from build123d import *

# Parameters (mm, degrees)
SKETCH2_W           = 127
SKETCH2_H           = 215.9
BASE_FLANGE1_DEPTH  = 0.7
EDGE_FLANGE4_DEPTH  = 127
EDGE_FLANGE5_DEPTH  = 216.9
EDGE_FLANGE6_DEPTH  = 216.9
EDGE_FLANGE7_DEPTH  = 25.4
EDGE_FLANGE9_DEPTH  = 25.4
EDGE_FLANGE10_DEPTH = 15.4
EDGE_FLANGE11_DEPTH = 15.4
SKETCH76_W          = 12.7
SKETCH76_H          = 12.7
TAB1_DEPTH          = 0.7
SKETCH79_W          = 12.7
SKETCH79_H          = 12.7
TAB2_DEPTH          = 0.7
SKETCH86_R          = 3.15
CUT_EXTRUDE3_DEPTH  = 253.866214627
SKETCH87_W          = 70.35
SKETCH87_H          = 12.7
CUT_EXTRUDE4_DEPTH  = 253.866214627
SKETCH88_R          = 25.4
CUT_EXTRUDE5_DEPTH  = 10
SKETCH90_R          = 25.4
CUT_EXTRUDE6_DEPTH  = 300.389111358


# Sheet-metal steps are written as plain solids
with BuildPart() as part:
    # Sketch2 → Base-Flange1 (new body)
    with BuildSketch(Plane(origin=(0, 0, 0), x_dir=(1, 0, 0), z_dir=(0, 1, 0))):
        Rectangle(SKETCH2_W, SKETCH2_H)
    extrude(amount=-BASE_FLANGE1_DEPTH)

    # Edge-Flange4 section (across the edge) → Edge-Flange4 (add)
    with BuildSketch(Plane(origin=(63.5, 0, -109.95), x_dir=(0, 0, 1), z_dir=(-1, 0, 0))):
        with BuildLine():
            Line((-0.7, 1), (-0.7, 177.8))
            Line((-0.7, 177.8), (0, 177.8))
            Line((0, 177.8), (0, 1))
            ThreePointArc((0, 1), (0.292893219, 0.292893219), (1, 0))
            Line((1, 0), (2, 0))
            Line((2, 0), (2, -0.7))
            Line((2, -0.7), (1, -0.7))
            ThreePointArc((1, -0.7), (-0.202081528, -0.202081528), (-0.7, 1))
        make_face()
    extrude(amount=EDGE_FLANGE4_DEPTH)

    # Edge-Flange5 section (across the edge) → Edge-Flange5 (add)
    with BuildSketch(Plane(origin=(-65.5, 0, -108.95), x_dir=(1, 0, 0), z_dir=(0, 0, 1))):
        with BuildLine():
            Line((-0.7, 1), (-0.7, 177.8))
            Line((-0.7, 177.8), (0, 177.8))
            Line((0, 177.8), (0, 1))
            ThreePointArc((0, 1), (0.292893219, 0.292893219), (1, 0))
            Line((1, 0), (2, 0))
            Line((2, 0), (2, -0.7))
            Line((2, -0.7), (1, -0.7))
            ThreePointArc((1, -0.7), (-0.202081528, -0.202081528), (-0.7, 1))
        make_face()
    extrude(amount=EDGE_FLANGE5_DEPTH)

    # Edge-Flange6 section (across the edge) → Edge-Flange6 (add)
    with BuildSketch(Plane(origin=(65.5, 0, 107.95), x_dir=(-1, 0, 0), z_dir=(0, 0, -1))):
        with BuildLine():
            Line((-0.7, 1), (-0.7, 177.8))
            Line((-0.7, 177.8), (0, 177.8))
            Line((0, 177.8), (0, 1))
            ThreePointArc((0, 1), (0.292893219, 0.292893219), (1, 0))
            Line((1, 0), (2, 0))
            Line((2, 0), (2, -0.7))
            Line((2, -0.7), (1, -0.7))
            ThreePointArc((1, -0.7), (-0.202081528, -0.202081528), (-0.7, 1))
        make_face()
    extrude(amount=EDGE_FLANGE6_DEPTH)

    # Edge-Flange7 section (across the edge) → Edge-Flange7 (add)
    with BuildSketch(Plane(origin=(-65.5, 127, -110.75), x_dir=(0, 0, 1), z_dir=(0, 1, 0))):
        with BuildLine():
            Line((-0.7, 1), (-0.7, 24.7))
            Line((-0.7, 24.7), (0, 24.7))
            Line((0, 24.7), (0, 1))
            ThreePointArc((0, 1), (0.292893219, 0.292893219), (1, 0))
            Line((1, 0), (1.8, 0))
            Line((1.8, 0), (1.8, -0.7))
            Line((1.8, -0.7), (1, -0.7))
            ThreePointArc((1, -0.7), (-0.202081528, -0.202081528), (-0.7, 1))
        make_face()
    extrude(amount=EDGE_FLANGE7_DEPTH)

    # Edge-Flange9 section (across the edge) → Edge-Flange9 (add)
    with BuildSketch(Plane(origin=(65.5, 152.4, -110.75), x_dir=(0, 0, 1), z_dir=(0, -1, 0))):
        with BuildLine():
            Line((-0.7, 1), (-0.7, 24.7))
            Line((-0.7, 24.7), (0, 24.7))
            Line((0, 24.7), (0, 1))
            ThreePointArc((0, 1), (0.292893219, 0.292893219), (1, 0))
            Line((1, 0), (1.8, 0))
            Line((1.8, 0), (1.8, -0.7))
            Line((1.8, -0.7), (1, -0.7))
            ThreePointArc((1, -0.7), (-0.202081528, -0.202081528), (-0.7, 1))
        make_face()
    extrude(amount=EDGE_FLANGE9_DEPTH)

    # Edge-Flange10 section (across the edge) → Edge-Flange10 (add)
    with BuildSketch(Plane(origin=(65.5, 25.4, 120.95), x_dir=(0, 0, -1), z_dir=(0, 1, 0))):
        with BuildLine():
            Line((-0.7, 1), (-0.7, 10))
            Line((-0.7, 10), (0, 10))
            Line((0, 10), (0, 1))
            ThreePointArc((0, 1), (0.292893219, 0.292893219), (1, 0))
            Line((1, 0), (13, 0))
            Line((13, 0), (13, -0.7))
            Line((13, -0.7), (1, -0.7))
            ThreePointArc((1, -0.7), (-0.202081528, -0.202081528), (-0.7, 1))
        make_face()
    extrude(amount=EDGE_FLANGE10_DEPTH)

    # Edge-Flange11 section (across the edge) → Edge-Flange11 (add)
    with BuildSketch(Plane(origin=(-65.5, 40.8, 120.95), x_dir=(0, 0, -1), z_dir=(0, -1, 0))):
        with BuildLine():
            Line((-0.7, 1), (-0.7, 10))
            Line((-0.7, 10), (0, 10))
            Line((0, 10), (0, 1))
            ThreePointArc((0, 1), (0.292893219, 0.292893219), (1, 0))
            Line((1, 0), (13, 0))
            Line((13, 0), (13, -0.7))
            Line((13, -0.7), (1, -0.7))
            ThreePointArc((1, -0.7), (-0.202081528, -0.202081528), (-0.7, 1))
        make_face()
    extrude(amount=EDGE_FLANGE11_DEPTH)

    # Sketch76 → Tab1 (add)
    with BuildSketch(Plane.ZY.offset(66.2)):
        with Locations((114.3, 8.35)):
            Rectangle(SKETCH76_W, SKETCH76_H)
    extrude(amount=-TAB1_DEPTH)

    # Sketch79 → Tab2 (add)
    with BuildSketch(Plane(origin=(66.2, 0, 0), x_dir=(0, 0, -1), z_dir=(1, 0, 0))):
        with Locations((-114.3, 8.35)):
            Rectangle(SKETCH79_W, SKETCH79_H)
    extrude(amount=-TAB2_DEPTH)

    # Sketch86 → Cut-Extrude3 (cut, through all)
    with BuildSketch(Plane(origin=(66.2, 0, 0), x_dir=(0, 0, -1), z_dir=(1, 0, 0))):
        with Locations(Location((-114.3, 8.35, 0), (0, 0, 90))):
            Circle(SKETCH86_R)
    extrude(amount=-CUT_EXTRUDE3_DEPTH, mode=Mode.SUBTRACT)

    # Sketch87 → Cut-Extrude4 (cut, through all)
    with BuildSketch(Plane.ZY.offset(66.2)):
        with Locations((-54.725, 165.1)):
            Rectangle(SKETCH87_W, SKETCH87_H)
        with Locations((53.725, 165.0975)):
            Rectangle(SKETCH87_W, SKETCH87_H)
    extrude(amount=-CUT_EXTRUDE4_DEPTH, mode=Mode.SUBTRACT)

    # Sketch88 → Cut-Extrude5 (cut)
    with BuildSketch(Plane(origin=(0, 0, 0), x_dir=(1, 0, 0), z_dir=(0, 1, 0))):
        with Locations(Location((-32.75, 70.85, 0), (0, 0, 270))):
            Circle(SKETCH88_R)
        with Locations(Location((32.75, 70.85, 0), (0, 0, 270))):
            Circle(SKETCH88_R)
        with Locations(Location((-32.75, 7.35, 0), (0, 0, 270))):
            Circle(SKETCH88_R)
        with Locations(Location((32.75, 7.35, 0), (0, 0, 270))):
            Circle(SKETCH88_R)
    extrude(amount=-CUT_EXTRUDE5_DEPTH, mode=Mode.SUBTRACT)

    # Sketch90 → Cut-Extrude6 (cut, through all)
    with BuildSketch(Plane.XY.offset(-109.95)):
        with Locations((-31.75, 39.1)):
            Circle(SKETCH90_R)
        with Locations((31.75, 39.1)):
            Circle(SKETCH90_R)
        with Locations((-31.75, 96.25)):
            Circle(SKETCH90_R)
        with Locations((31.75, 96.25)):
            Circle(SKETCH90_R)
        with Locations((0, 146.05)):
            Circle(SKETCH90_R)
    extrude(amount=-CUT_EXTRUDE6_DEPTH, mode=Mode.SUBTRACT)


solid = part.part
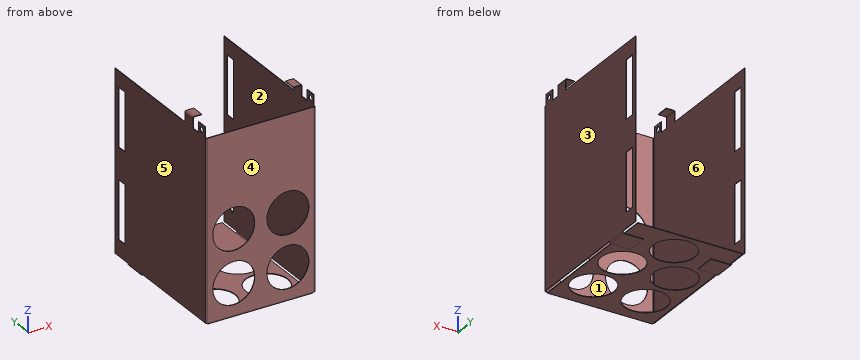
Model file for the job. Use its own axes, mm. Face numbers are marked on the shaded views. A direction names the side the tool comes from. Give positions to 0.01 mm unless a question says otherwise; leave off trailing zeros. Order: outer loops, then holes, each group sorted by start corner. A loop starts at its lowest first (then second) coordinate and runs counter-clockwise, first axis right, second up. Notation, with made-up numbers: (62, -39) - (90, -39) arc R27 cw to (90, -15) - close; hole circle Ø10 at (36.5, 36). An arc over 180 degrees is marked (long way). One line per item, written item: value.
Item 1: Wall check: line 1 (Y direction, x = -31.75, z = -110.3); line 2 (Z direction, x = 60, y = 38.5); line 3 (X direction, y = 50, z = -96). Give the ranges that are in metal, low to high.
Response values:
line 1: -0.03 to 13.7, 64.5 to 70.85, 121.65 to 177.8
line 2: -110.65 to -109.95, 120.95 to 121.65
line 3: -66.2 to -65.5, 65.5 to 66.2
Item 2: Slice it at D-D (x = 32.75). List the corners of the cut face in (y, z).
Response values:
outline: (-0.7, -108.95) arc R1.7 ccw to (1, -110.65) - (13.72, -110.65) - (13.72, -109.95) - (1, -109.95) arc R1 cw to (0, -108.95) - (0, -96.25) - (-0.7, -96.25) - close; (-0.7, -45.45) - (0, -45.45) - (0, -32.75) - (-0.7, -32.75) - close; (-0.7, 18.05) - (0, 18.05) - (0, 107.95) - (-0.7, 107.95) - close; (64.48, -110.65) - (70.87, -110.65) - (70.87, -109.95) - (64.48, -109.95) - close; (121.63, -110.65) - (177.8, -110.65) - (177.8, -109.95) - (121.63, -109.95) - close
Item 3: Pin check, flat tips, straight feed: pin 1 Ø0.8 at (x, z) = (57, -109.5) entering from -Y; pin 2 Ø5 at (x, z) = (47, 45) entering from +Y; pin 3 Ø5 at (y, z) = (8.35, 114.3) entering from -X; pin 4 Ø4.5 at (x, y) = (-58.5, 32) entering from -Z. Stop position of each tip, or through.
Response values:
pin 1: y = -0.69
pin 2: y = 0
pin 3: through
pin 4: z = -110.65
Item 4: Two-plate mould, pull along X, no slides. Class the marked faces 4, 5 and 6: released by +X, released by -X, zero draft, split by the parting line, or undercut.
Response values:
face 4: zero draft
face 5: released by -X
face 6: undercut
Item 5: Slice it at C-C (x = -10). List the corners of the cut face in (y, z).
Response values:
outline: (-0.7, -108.95) arc R1.7 ccw to (1, -110.65) - (25.98, -110.65) - (25.98, -109.95) - (1, -109.95) arc R1 cw to (0, -108.95) - (0, -82.15) - (-0.7, -82.15) - close; (-0.7, -59.55) - (0, -59.55) - (0, -18.65) - (-0.7, -18.65) - close; (-0.7, 3.95) - (0, 3.95) - (0, 107.95) - (-0.7, 107.95) - close; (52.22, -110.65) - (83.13, -110.65) - (83.13, -109.95) - (52.22, -109.95) - close; (109.37, -110.65) - (122.7, -110.65) - (122.7, -109.95) - (109.37, -109.95) - close; (169.4, -110.65) - (177.8, -110.65) - (177.8, -109.95) - (169.4, -109.95) - close
Item 6: Slice it at B-B (y = 8.35). List the corners of the cut face in (x, z).
Response values:
outline: (-66.2, -108.95) - (-65.5, -108.95) - (-65.5, 111.15) - (-66.2, 111.15) - close; (-66.2, 117.45) - (-65.5, 117.45) - (-65.5, 120.65) - (-66.2, 120.65) - close; (-63.5, -110.65) - (63.5, -110.65) - (63.5, -109.95) - (-63.5, -109.95) - close; (65.5, -108.95) - (66.2, -108.95) - (66.2, 111.15) - (65.5, 111.15) - close; (65.5, 117.45) - (66.2, 117.45) - (66.2, 120.65) - (65.5, 120.65) - close
Item 7: Tool access for the marked faces 1, 2 and 3: list every direction of +Z, -Z, +X, -X, +Y, -Y with a clear straight run to the whole face (end or side of a thin tool).
Response values:
face 1: +Z, +Y
face 2: +Y
face 3: +Z, -Z, +X, +Y, -Y
Item 8: Slice it at A-A (z = 57). List the corners of the cut face in (x, y), then the cut area to 3 significant figures.
Response values:
outline: (-66.2, 1) arc R1.7 ccw to (-64.5, -0.7) - (64.5, -0.7) arc R1.7 ccw to (66.2, 1) - (66.2, 158.75) - (65.5, 158.75) - (65.5, 1) arc R1 cw to (64.5, 0) - (-64.5, 0) arc R1 cw to (-65.5, 1) - (-65.5, 158.75) - (-66.2, 158.75) - close; (-66.2, 171.45) - (-65.5, 171.45) - (-65.5, 177.8) - (-66.2, 177.8) - close; (65.5, 171.45) - (66.2, 171.45) - (66.2, 177.8) - (65.5, 177.8) - close
area: 323 mm2
